from build123d import *

# Parameters (mm, degrees)
F1_DEPTH = 15
F3_DEPTH = 43.4455230334
F5_D     = 4
F6_R     = 5


with BuildPart() as f1:
    # F0 (on Front) → F1 (new body, symmetric)
    with BuildSketch(Plane.XZ):
        Polygon((50, 0), (0, 0), (0, -8), (46.2695387348, -8), (76.0110249394, -43.4445230334), (82.1393804843, -38.3022221559), align=None)
    extrude(amount=F1_DEPTH, both=True)

    # F2 (on face) → F3 (cut, through all)
    with BuildSketch(Plane.XY):
        with BuildLine():
            ThreePointArc((17.4500849098, 3), (14.4500849098, 0), (17.4500849098, -3))
            Line((17.4500849098, -3), (37.4500849098, -3))
            ThreePointArc((37.4500849098, -3), (40.4500849098, 0), (37.4500849098, 3))
            Line((37.4500849098, 3), (17.4500849098, 3))
        make_face()
    extrude(amount=-F3_DEPTH, mode=Mode.SUBTRACT)

    # F5 (through all)
    with Locations(Plane(origin=(29.3412044417, 0, 24.6201938253), x_dir=(0, 1, 0), z_dir=(0.7660444431, 0, 0.6427876097))):
        with Locations((0, -47.1393804843), (0, -67.1393804843)):
            Hole(F5_D / 2)

    # F6
    f6_edges = [f1.edges().sort_by_distance(p)[0] for p in [
        (79.075203, -15, -40.873373),
        (79.075203, 15, -40.873373),
        (0, 15, -4),
        (0, -15, -4),
    ]]
    fillet(f6_edges, radius=F6_R)


solid = f1.part
Check sheet for the modelled part. Datum: model origin and axes. Units: mm. A direction names the side the tool comes from. Round coordinates to 2 decimals unless told otherwise and drop trailing zeros. Order: outer loops, then holes, each group sorted by start corner. A loop starts at its lowest first (then second) coordinate and runs counter-clockwise, first axis right, second up.
Q1. Cross-section at B-B, the plane z = -5.5. Enter the section's corners in (x, y).
Filled sheet:
outline: (0, -10) arc R5 ccw to (5, -15) - (54.62, -15) - (54.62, 15) - (5, 15) arc R5 ccw to (0, 10) - close; hole (17.45, -3) - (37.45, -3) arc R3 ccw to (37.45, 3) - (17.45, 3) arc R3 ccw to start
Q2. Draft check along X on faces 1 (the face through (47, -15, -8)), 2 (the face through (78.15, 13.57, -39.69)), 3 (the face through (28, 3, -4)). Enter one of: pulls with the +X half, pulls with the -X half, needs draft (parallel to the pull), parting line crosses it, or undercut.
Filled sheet:
face 1: needs draft
face 2: pulls with the +X half
face 3: undercut
Q3. Cross-section at C-C, the plane y = -6. Enter the section's corners in (x, z).
Filled sheet:
outline: (0, -8) - (46.27, -8) - (76.01, -43.44) - (82.14, -38.3) - (50, 0) - (0, 0) - close
Q4. Set-up check for faces 4 (the face through (23, -4, -8)), 5 (the face through (14.45, 0.07, -3.94)), 6 (the face through (25, -4, 0)): record each of +Z, -Z, +X, -X, +Y, -Y from which the full face is reachable in a straight line by a thin tool's end or side.
Filled sheet:
face 4: -Z, -X, +Y, -Y
face 5: +Z, -Z
face 6: +Z, +X, -X, +Y, -Y
Q5. Scan lines: L1, parallel to X at y = -2, z = -2; L2, parallel to Z at x = 35, y = 11; L3, parallel to X at y = -4, z = -21.5. Record each from-to range of solid material in increasing order.
Filled sheet:
L1: x = 0 to 15.21, 39.69 to 51.68
L2: z = -8 to 0
L3: x = 57.6 to 68.04
Q6. Cross-section at A-A, the plane x = 35. Enter the section's corners in (y, z), plus the area to 3 significant figures.
Filled sheet:
outline: (-15, -8) - (-3, -8) - (-3, 0) - (-15, 0) - close; (3, -8) - (15, -8) - (15, 0) - (3, 0) - close
area: 192 mm2
Q7. Cross-section at D-D, the plane y = 0. Enter the section's corners in (x, z).
Filled sheet:
outline: (0, -8) - (14.45, -8) - (14.45, 0) - (0, 0) - close; (40.45, -8) - (46.27, -8) - (52.23, -15.1) - (58.36, -9.96) - (50, 0) - (40.45, 0) - close; (54.8, -18.17) - (65.08, -30.42) - (71.21, -25.28) - (60.93, -13.02) - close; (67.65, -33.49) - (76.01, -43.44) - (82.14, -38.3) - (73.78, -28.34) - close
Q8. Depth check by flat-ended pin: P1, Ø1.5, axis at x = 9.5, y = -3.5, coming from the -Z side; P2, Ø5, axis at x = 69, y = 4, coming from the +Z side; P3, Ø3, axis at y = 4.5, z = -39, coming from the -X side; P4, Ø6, axis at x = 44.5, z = -14, coming from the +Y side. Enter the tip coordinate at first touch or a pass-through.
Filled sheet:
P1: stops at z = -8
P2: stops at z = -19.66
P3: stops at x = 71.02
P4: passes through
